Geometry: final body of the model. Coordinates: model frame, mm. A direction names the side the tool comes from. Give positions to 0.01 mm unless a question says otherwise; leave off trailing zeros. Write each loop counter-clockwise with the first axis right and the second up, starting at its lowest first coordinate (ties: lowest second). Pieces come first, ordered by that corner, then holes.
```python
from build123d import *

# Parameters (mm, degrees)
PER_AGE1_D              = 10
PER_AGE1_DEPTH          = 20.5
PER_AGE1_TIP            = 3.004303095
ESQUISSE4_OUTSIDE_W     = 51.064
ESQUISSE4_OUTSIDE_H     = 51.064
ENL_V_MAT_EXTRU_2_DEPTH = 13.500004827


with BuildPart() as part:
    # Esquisse1 → Base-Révolution (revolve)
    with BuildSketch(Plane.XY, mode=Mode.PRIVATE) as base_r_volution_sk:
        with BuildLine():
            Line((0, 17.5), (0, 18.5))
            Line((0, 18.5), (8, 18.5))
            Line((8, 18.5), (8, 17.5))
            Line((8, 17.5), (8.313200902, 17.5))
            ThreePointArc((8.313200902, 17.5), (8.879337334, 17.324311555), (9.246546508, 16.858979079))
            Line((9.246546508, 16.858979079), (10.446259113, 13.739726306))
            ThreePointArc((10.446259113, 13.739726306), (11.997253194, 11.624097191), (14.405880363, 10.584874234))
            Line((14.405880363, 10.584874234), (24.641421356, 9.122654092))
            ThreePointArc((24.641421356, 9.122654092), (25.255453955, 8.78790634), (25.5, 8.132704598))
            Line((25.5, 8.132704598), (25.5, 0))
            Line((25.5, 0), (-4.5, 0))
            ThreePointArc((-4.5, 0), (-3.799049548, 8.364652706), (-1.708679537, 16.494172966))
            ThreePointArc((-1.708679537, 16.494172966), (-1.160964211, 17.222959412), (-0.292419293, 17.5))
            Line((-0.292419293, 17.5), (0, 17.5))
        make_face()
    revolve(base_r_volution_sk.sketch.rotate(Axis((95.260513245, 0, 0), (-1, 0, 0)), 90), axis=Axis((95.260513245, 0, 0), (-1, 0, 0)))  # turned: the seam where the file's is

    # Perçage1
    with Locations(Plane(origin=(25.5, 0, 0), x_dir=(0, 0, -1), z_dir=(1, 0, 0))):
        with Locations((0, 0)):
            Hole(PER_AGE1_D / 2, depth=PER_AGE1_DEPTH)
            with Locations((0, 0, -(PER_AGE1_DEPTH + PER_AGE1_TIP / 2))):  # 118° drill point
                Cone(0, PER_AGE1_D / 2, PER_AGE1_TIP, mode=Mode.SUBTRACT)

    # Esquisse4 outside → Enlèv. mat.-Extru.2 (cut, through all)
    with BuildSketch(Plane(origin=(8, 0, 0), x_dir=(0, 0, -1), z_dir=(1, 0, 0))):
        Rectangle(ESQUISSE4_OUTSIDE_W, ESQUISSE4_OUTSIDE_H)
        with BuildLine():
            ThreePointArc((-17.957142857, 0.889393281), (-18.5, 0), (-17.957142857, -0.889393281))
            ThreePointArc((-17.957142857, -0.889393281), (-17.418918919, -1.682635937), (-17.79535636, -2.564233221))
            ThreePointArc((-17.79535636, -2.564233221), (-18.157937121, -3.541090159), (-17.454878328, -4.310130223))
            ThreePointArc((-17.454878328, -4.310130223), (-16.774965689, -4.985031065), (-16.974612988, -5.922001341))
            ThreePointArc((-16.974612988, -5.922001341), (-17.143103155, -6.954423684), (-16.302302488, -7.576789389))
            ThreePointArc((-16.302302488, -7.576789389), (-15.508197398, -8.108380814), (-15.527199047, -9.063802853))
            ThreePointArc((-15.527199047, -9.063802853), (-15.497610903, -10.103170336), (-14.559029214, -10.55063501))
            ThreePointArc((-14.559029214, -10.55063501), (-13.67429749, -10.920787188), (-13.507953431, -11.865293679))
            ThreePointArc((-13.507953431, -11.865293679), (-13.535960556, -12.405745053), (-13.278297709, -12.881646244))
            ThreePointArc((-13.278297709, -12.881646244), (0, -18.5), (13.278297709, -12.881646244))
            ThreePointArc((13.278297709, -12.881646244), (13.535960556, -12.405745053), (13.507953431, -11.865293679))
            ThreePointArc((13.507953431, -11.865293679), (13.67429749, -10.920787188), (14.559029214, -10.55063501))
            ThreePointArc((14.559029214, -10.55063501), (15.497610903, -10.103170336), (15.527199047, -9.063802853))
            ThreePointArc((15.527199047, -9.063802853), (15.508197398, -8.108380814), (16.302302488, -7.576789389))
            ThreePointArc((16.302302488, -7.576789389), (17.143103155, -6.954423684), (16.974612988, -5.922001341))
            ThreePointArc((16.974612988, -5.922001341), (16.774965689, -4.985031065), (17.454878328, -4.310130223))
            ThreePointArc((17.454878328, -4.310130223), (18.157937121, -3.541090159), (17.79535636, -2.564233221))
            ThreePointArc((17.79535636, -2.564233221), (17.418918919, -1.682635937), (17.957142857, -0.889393281))
            ThreePointArc((17.957142857, -0.889393281), (18.5, 0), (17.957142857, 0.889393281))
            ThreePointArc((17.957142857, 0.889393281), (17.418918919, 1.682635937), (17.79535636, 2.564233221))
            ThreePointArc((17.79535636, 2.564233221), (18.157937121, 3.541090159), (17.454878328, 4.310130223))
            ThreePointArc((17.454878328, 4.310130223), (16.774965689, 4.985031065), (16.974612988, 5.922001341))
            ThreePointArc((16.974612988, 5.922001341), (17.143103155, 6.954423684), (16.302302488, 7.576789389))
            ThreePointArc((16.302302488, 7.576789389), (15.508197398, 8.108380814), (15.527199047, 9.063802853))
            ThreePointArc((15.527199047, 9.063802853), (15.497610903, 10.103170336), (14.559029214, 10.55063501))
            ThreePointArc((14.559029214, 10.55063501), (13.67429749, 10.920787188), (13.507953431, 11.865293679))
            ThreePointArc((13.507953431, 11.865293679), (13.535960556, 12.405745053), (13.278297709, 12.881646244))
            ThreePointArc((13.278297709, 12.881646244), (0, 18.5), (-13.278297709, 12.881646244))
            ThreePointArc((-13.278297709, 12.881646244), (-13.535960556, 12.405745053), (-13.507953431, 11.865293679))
            ThreePointArc((-13.507953431, 11.865293679), (-13.67429749, 10.920787188), (-14.559029214, 10.55063501))
            ThreePointArc((-14.559029214, 10.55063501), (-15.497610903, 10.103170336), (-15.527199047, 9.063802853))
            ThreePointArc((-15.527199047, 9.063802853), (-15.508197398, 8.108380814), (-16.302302488, 7.576789389))
            ThreePointArc((-16.302302488, 7.576789389), (-17.143103155, 6.954423684), (-16.974612988, 5.922001341))
            ThreePointArc((-16.974612988, 5.922001341), (-16.774965689, 4.985031065), (-17.454878328, 4.310130223))
            ThreePointArc((-17.454878328, 4.310130223), (-18.157937121, 3.541090159), (-17.79535636, 2.564233221))
            ThreePointArc((-17.79535636, 2.564233221), (-17.418918919, 1.682635937), (-17.957142857, 0.889393281))
        make_face(mode=Mode.SUBTRACT)
    extrude(amount=-ENL_V_MAT_EXTRU_2_DEPTH, mode=Mode.SUBTRACT)


solid = part.part
```
Item 1: Section A-A, the plane x = 16. Return the cut outline in (y, z).
Found:
outline: circle Ø20.71 at (0, 0); hole circle Ø10 at (0, 0)
Item 2: Line query: L1, parallel to Z at x = 6.5, y = -0.5; L2, parallel to Y at x = 20, z = 0; L3, parallel to Y at x = 10.5, z = 1. Output: solid intervals per line, ascending.
Found:
L1: z = -18.37 to -4.97, 4.97 to 18.37
L2: y = -9.79 to -5, 5 to 9.79
L3: y = -13.57 to -4.9, 4.9 to 13.57
Item 3: Pin query (flat end, axial travel): pin 1 Ø1 at (y, z) = (9, 15) entering from -X; pin 2 Ø0.7 at (y, z) = (-3, -17) entering from -X; pin 3 Ø0.9 at (y, z) = (-6.5, -16.5) entering from +X; pin 4 Ø5 at (x, z) = (21.5, -14.5) entering from -Y. Return the tip coordinate at first contact, or that it passes through.
Found:
pin 1: stops at x = -1.42
pin 2: stops at x = -1.48
pin 3: stops at x = 8.93
pin 4: passes through
Item 4: Section B-B, the plane x = 23. Return the cut outline in (y, z), plus the area to 3 significant figures.
Found:
outline: circle Ø18.71 at (0, 0); hole circle Ø10 at (0, 0)
area: 197 mm2
Item 5: Pull-direction query (Y, two-part tool) for faces 1 (the face through (4.1, -10.1, -15.5)), 2 (the face through (25.5, -4, -4)); classes: +Y half, -Y half, draft (parallel to the pull), parting line (faces both ways), or undercut.
Found:
face 1: undercut
face 2: draft
Item 6: Reachability of faces 3 (the face through (8, 10, -15)), 4 (the face through (0, -6.7, 16.5)), 5 (the face through (8, -10, -15)), 6 (the face through (0, 18, 1)) from +Z, -Z, +X, -X, +Y, -Y: full face, straight path, thin tool, end or side. Return the list, or none.
Found:
face 3: -Z, +X, +Y
face 4: +Z, -X, -Y
face 5: -Z, +X, -Y
face 6: -X, +Y
